Can you work these out from the model? Positions are in its coordinate system, mm. Give positions to 0.01 mm unless a question says otherwise; leave off trailing zeros. Write each loop counter-clockwise with the first axis right and the second up, starting at its lowest first coordinate (ties: lowest second). Pieces come first, ordered by that corner, then holes.
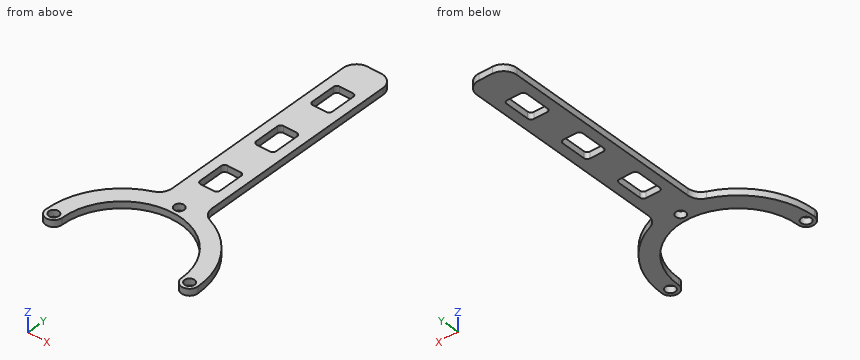
from build123d import *

# Parameters (mm, degrees)
SKETCH_1_W      = 6
SKETCH_1_H      = 9.5
SKETCH_1_R      = 1.5
EXTRUDE_1_DEPTH = 2
FILLET_1_R      = 1
FILLET_2_R      = 4


with BuildPart() as part:
    # 草图1 → 凸台-拉伸1 (new body)
    with BuildSketch(Plane.XY):
        with BuildLine():
            Line((6, 22.203603311), (6, 90))
            Line((6, 90), (-6, 90))
            Line((-6, 90), (-6, 22.203603311))
            ThreePointArc((-6, 22.203603311), (-18.261982368, 13.982131454), (-23, 0))
            ThreePointArc((-23, 0), (-20.5, -2.5), (-18, 0))
            ThreePointArc((-18, 0), (0, 18), (18, 0))
            ThreePointArc((18, 0), (20.5, -2.5), (23, 0))
            ThreePointArc((23, 0), (18.261982368, 13.982131454), (6, 22.203603311))
        make_face()
        with Locations((0, 35.25)):
            Rectangle(SKETCH_1_W, SKETCH_1_H, mode=Mode.SUBTRACT)
        with Locations((0, 55.25)):
            Rectangle(SKETCH_1_W, SKETCH_1_H, mode=Mode.SUBTRACT)
        with Locations((0, 75.25)):
            Rectangle(SKETCH_1_W, SKETCH_1_H, mode=Mode.SUBTRACT)
        with Locations((0, 20.5)):
            Circle(SKETCH_1_R, mode=Mode.SUBTRACT)
        with Locations((20.5, 0)):
            Circle(SKETCH_1_R, mode=Mode.SUBTRACT)
        with Locations((-20.5, 0)):
            Circle(SKETCH_1_R, mode=Mode.SUBTRACT)
    extrude(amount=EXTRUDE_1_DEPTH)

    # 圆角1
    fillet_1_edges = [part.edges().sort_by_distance(p)[0] for p in [
        (3, 30.5, 1),
        (3, 40, 1),
        (-3, 40, 1),
        (-3, 30.5, 1),
        (3, 50.5, 1),
        (3, 60, 1),
        (-3, 60, 1),
        (-3, 50.5, 1),
        (-3, 80, 1),
        (-3, 70.5, 1),
        (3, 70.5, 1),
        (3, 80, 1),
    ]]
    fillet(fillet_1_edges, radius=FILLET_1_R)

    # 圆角2
    fillet_2_edges = [part.edges().sort_by_distance(p)[0] for p in [
        (-6, 22.203603311, 1),
        (-6, 90, 1),
        (6, 90, 1),
        (6, 22.203603311, 1),
    ]]
    fillet(fillet_2_edges, radius=FILLET_2_R)


solid = part.part
(1) Imagine slicing it at C-C, the plane x = -20. Write out the boundary of the cut face in (y, z).
Returned:
outline: (-2.45, 0) - (-1.41, 0) - (-1.41, 2) - (-2.45, 2) - close; (1.41, 0) - (11.36, 0) - (11.36, 2) - (1.41, 2) - close
(2) Imagine slicing it at D-D, the plane z = 0.85. Give the number of separate pieces and of enclosed holes in the cut face, plus the area to 3 significant figures.
Returned:
separate pieces: 1
enclosed holes: 6
area: 955 mm2
(3) Imagine slicing it at A-A, the plane x = 0. Write out the boundary of the cut face in (y, z).
Returned:
outline: (18, 0) - (19, 0) - (19, 2) - (18, 2) - close; (22, 0) - (30.5, 0) - (30.5, 2) - (22, 2) - close; (40, 0) - (50.5, 0) - (50.5, 2) - (40, 2) - close; (60, 0) - (70.5, 0) - (70.5, 2) - (60, 2) - close; (80, 0) - (90, 0) - (90, 2) - (80, 2) - close
(4) Imagine slicing it at B-B, the plane y = 36.5. Write out the boundary of the cut face in (x, z).
Returned:
outline: (-6, 0) - (-3, 0) - (-3, 2) - (-6, 2) - close; (3, 0) - (6, 0) - (6, 2) - (3, 2) - close
(5) If I drill on L1, parallel to Y at x = 0, z = 1.65; L2, parallel to X at y = 76, z = 0.4; L3, parallel to X at y = 45.5, z = 1.35, over which ranges is the centre line in solid material (lowest first)?
Returned:
L1: y = 18 to 19, 22 to 30.5, 40 to 50.5, 60 to 70.5, 80 to 90
L2: x = -6 to -3, 3 to 6
L3: x = -6 to 6
(6) Will these pins go through, and if not, where does the flat tip stop? P1, Ø1, axis at x = 11, z = 1, coming from the -Y side; P2, Ø1, axis at y = 75, z = 1.5, coming from the -X side.
Returned:
P1: stops at y = 13.85
P2: stops at x = -6
